Part print with two shaded views. Sizes in mm from the minimum x, y, z corner. A direction names the side the tool comes from. Give positions to 0.01 mm unless a question says otherwise; leave off trailing zeros. Order: outer loops, then holes, each group sorted by start corner. A loop starts at its lowest first (then second) coordinate and runs counter-clockwise, first axis right, second up. Notation, with made-up numbers: M 43,13.5 L 91,13.5 A26 ccw 91,43.5 Z; hole C -4,67.5 d7. An arc over 180 degrees is marked long. Write each question's results on one line, items separated by ' | '. Start each with the question number.
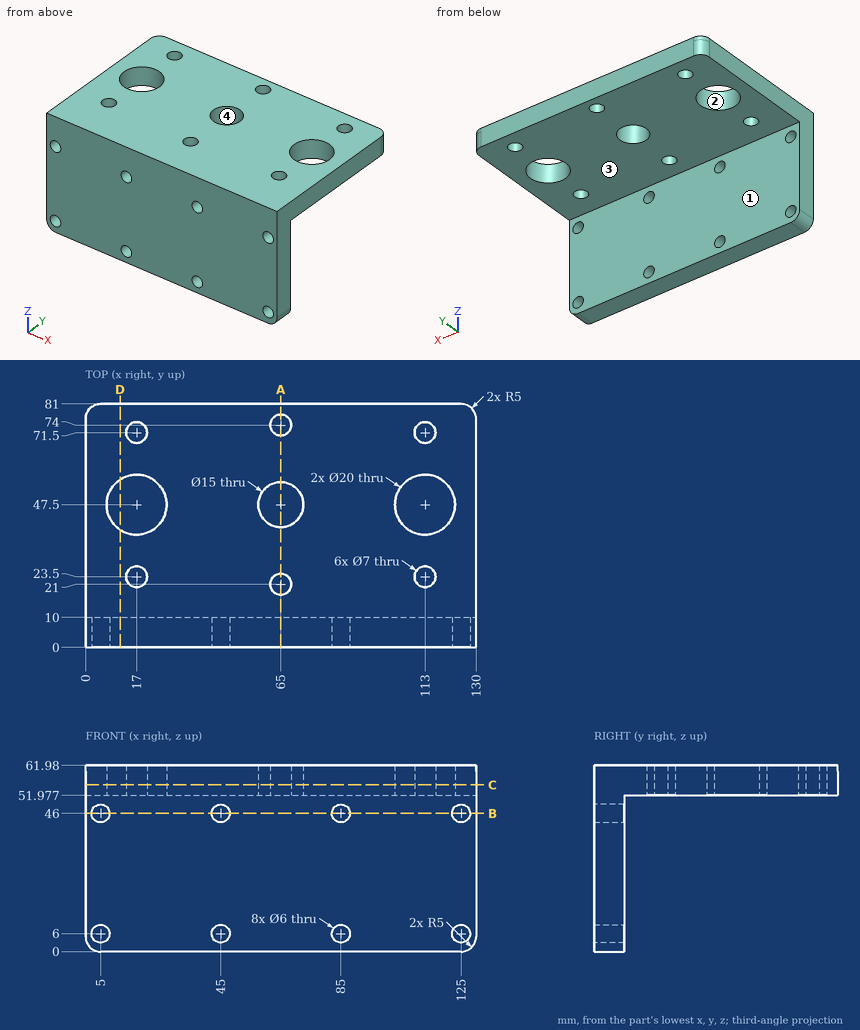
(1) Tool access for the marked faces 1 and 2: list every direction of +Z, -Z, +X, -X, +Y, -Y with a clear straight run to the whole face (end or side of a thin tool).
(2) Drop flat-ended pins along their axis: P1, Ø8, axis at x = 45, z = 6, coming from the +Y side; P2, Ø10, axis at x = 36, y = 71, coming from the -Z side; P3, Ø18, axis at x = 17, y = 47.5, coming from the -Z side. Give the stop position or say it passes through.
(3) Saw through at A-A on x = 65. Give the cut face in (y, z), plus the area to 3 significant figures.
(4) Probe L1, parallel to X at y = 5, z = 6; L2, parallel to Z at x = 85, y = 8; L3, parallel to Y at x = 65, z = 59. List the from-to ranges inside material, lowest first.
(5) Saw through at C-C on z = 55.5. Give the number of separate pieces and of enclosed holes in the cut face, plus the area to 3 significant figures.
(6) Saw through at D-D on x = 11.5. Give the cut face in (y, z), plus the area to 3 significant figures.
(7) Pull direction X, two halves, no side cores. Call the marked faces 3 and 4: +X half, -X half, draft (parallel to the pull), parting line (faces both ways), or undercut.
(8) Saw through at B-B on z = 46. Give the cut face in (x, y), plus the area to 3 significant figures.
Taken from the geometry:
1) face 1: -Z, +X, -X, +Y | face 2: +Z, -Z
2) P1: stops at y = 10 | P2: stops at z = 51.98 | P3: passes through
3) outline: M 0,0 L 10,0 L 10,51.98 L 17.5,51.98 L 17.5,61.98 L 0,61.98 Z; M 24.5,51.98 L 40,51.98 L 40,61.98 L 24.5,61.98 Z; M 55,51.98 L 70.5,51.98 L 70.5,61.98 L 55,61.98 Z; M 77.5,51.98 L 81,51.98 L 81,61.98 L 77.5,61.98 Z | area: 1,040 mm²
4) L1: x = 0 to 2, 8 to 42, 48 to 82, 88 to 122, 128 to 130 | L2: z = 0 to 3, 9 to 43, 49 to 61.98 | L3: y = 0 to 17.5, 24.5 to 40, 55 to 70.5, 77.5 to 81
5) separate pieces: 1 | enclosed holes: 9 | area: 9,480 mm²
6) outline: M 0,0 L 10,0 L 10,51.98 L 39.15,51.98 L 39.15,61.98 L 0,61.98 Z; M 55.85,51.98 L 81,51.98 L 81,61.98 L 55.85,61.98 Z | area: 1,160 mm²
7) face 3: draft | face 4: undercut
8) outline: M 0,0 L 2,0 L 2,10 L 0,10 Z; M 8,0 L 42,0 L 42,10 L 8,10 Z; M 48,0 L 82,0 L 82,10 L 48,10 Z; M 88,0 L 122,0 L 122,10 L 88,10 Z; M 128,0 L 130,0 L 130,10 L 128,10 Z | area: 1,060 mm²
